Geometry: see drawing. Coordinates: mm, zero at the bounding-box minimum. A direction names the side the tool comes from. Give positions to 0.01 mm unless a question says otherwise; leave off trailing zeros. Write each loop counter-clockwise with the first axis right and the second up, starting at its lowest first coordinate (ties: lowest second). Pieces come first, ordered by that corner, then holes. Notation, with made-up numbers: (15.25, 70) -> (48.25, 70) arc R27 ccw to (48.25, 86) -> close; hole circle Ø7 at (31.25, -23). An arc over 180 degrees is marked (long way). Answer as a JSON object with one key per item and string values. Group by question number.
Item 1: Access query for the marked faces 1 and 2. Directions: +Z, -Z, +X, -X, +Y, -Y. A direction counts if a zero-diameter tool reaches every point of the face in a straight line with its end or side. Return the directions, or none.
Item 2: Ray query, probe 1 along X at (y, z) = (197.5, 253.5); probe 2 along Z at (x, y) = (291, 215); probe 3 along Z at (x, y) = (197, 25.5). Return the intervals inside material, ascending. Write a range as from..to.
Item 3: Section query C-C on x = 268.5. Return the cut outline in (y, z), plus the area to 3 significant figures.
Item 4: Section query A-A on z = 200. Return the cut outline in (x, y).
Item 5: Section query B-B on y = 200. Return the cut outline in (x, z).
Item 6: First-contact query: pin 1 Ø5 at (x, z) = (320.5, 255.5) entering from -Y; pin 2 Ø10 at (x, z) = (230, 130.5) entering from -Y; pin 3 Ø24 at (y, z) = (80.5, 360) entering from +X. Flat tips, straight axial feed; report the tip coordinate or a pass-through.
Item 7: Section query D-D on y = 59. Return the cut outline in (x, z).
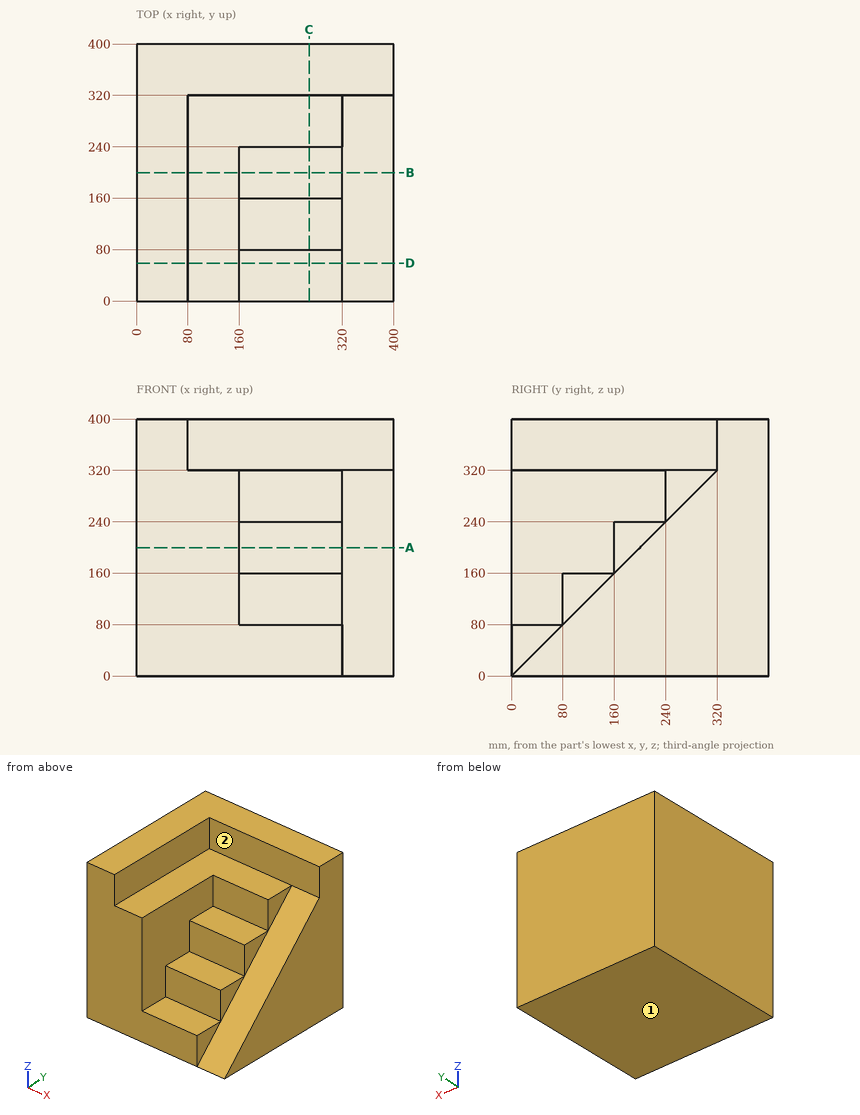
Worked answers:
{
 "1": {"face 1": "-Z, +X, -X, +Y, -Y", "face 2": "+Z, +X, -Y"},
 "2": {"probe 1": "0..160", "probe 2": "0..240", "probe 3": "0..80"},
 "3": {"outline": "(0, 0) -> (400, 0) -> (400, 400) -> (320, 400) -> (320, 320) -> (240, 320) -> (240, 240) -> (160, 240) -> (160, 160) -> (80, 160) -> (80, 80) -> (0, 80) -> close", "area": "96,000 mm^2"},
 "4": {"outline": "(0, 0) -> (160, 0) -> (160, 160) -> (320, 160) -> (320, 200) -> (400, 200) -> (400, 400) -> (0, 400) -> close"},
 "5": {"outline": "(0, 0) -> (400, 0) -> (400, 200) -> (320, 200) -> (320, 240) -> (160, 240) -> (160, 320) -> (80, 320) -> (80, 400) -> (0, 400) -> close"},
 "6": {"pin 1": "y = 240", "pin 2": "y = 80", "pin 3": "x = 80"},
 "7": {"outline": "(0, 0) -> (400, 0) -> (400, 59) -> (320, 59) -> (320, 80) -> (160, 80) -> (160, 320) -> (80, 320) -> (80, 400) -> (0, 400) -> close"}
}
